Design review of the part built by this model. Coordinates are the model's own, in mm. A direction names the side the tool comes from. Give positions to 0.01 mm unless a question says otherwise; leave off trailing zeros. Loops run counter-clockwise (first coordinate to the right, second up) from the corner with the lowest first, then second, coordinate; pieces in that order, holes last.
from build123d import *

# Parameters (mm, degrees)
SKIZZE1_W                       = 21.5
SKIZZE1_H                       = 17
AUFSATZ_LINEAR_AUSTRAGEN1_DEPTH = 1
VERRUNDUNG1_R                   = 0.5
SCHNITT_LINEAR_AUSTRAGEN1_REACH = 25.141
SKIZZE4_W                       = 3
SKIZZE4_H                       = 0.25
SCHNITT_LINEAR_AUSTRAGEN2_DEPTH = 1
VERRUNDUNG2_R                   = 0.5
SCHNITT_LINEAR_AUSTRAGEN3_DEPTH = 1
SCHNITT_LINEAR_START            = -1
SCHNITT_LINEAR_AUSTRAGEN4_DEPTH = 1


with BuildPart() as part:
    # Skizze1 → Aufsatz-Linear austragen1 (new body)
    with BuildSketch(Plane(origin=(0, 0, 0), x_dir=(1, 0, 0), z_dir=(0, 1, 0))):
        Rectangle(SKIZZE1_W, SKIZZE1_H)
    extrude(amount=AUFSATZ_LINEAR_AUSTRAGEN1_DEPTH)

    # Verrundung1
    verrundung1_edges = [part.edges().sort_by_distance(p)[0] for p in [
        (-10.75, 1, 0),
        (10.75, 1, 0),
        (0, 1, -8.5),
    ]]
    fillet(verrundung1_edges, radius=VERRUNDUNG1_R)

    # Schnitt-Linear austragen1: up to this face of the body (flat: up to its plane)
    schnitt_linear_austragen1_end = Plane(part.part.faces().sort_by_distance((10.75, 0.25, 0))[0])
    # Skizze2 → Schnitt-Linear austragen1 (cut, up to the picked face)
    with BuildSketch(Plane.ZY.offset(10.75), mode=Mode.PRIVATE) as schnitt_linear_austragen1_sk1:
        Polygon((8.5, 0), (7.75, 1), (8.5, 1), align=None)
    schnitt_linear_austragen1_tool1 = split(extrude(schnitt_linear_austragen1_sk1.sketch, amount=-SCHNITT_LINEAR_AUSTRAGEN1_REACH, mode=Mode.PRIVATE), bisect_by=schnitt_linear_austragen1_end, keep=Keep.BOTH, mode=Mode.PRIVATE)
    add(schnitt_linear_austragen1_tool1.solids().sort_by(Axis((-10.75, 0.666667, 8.25), (1, 0, 0)))[0], mode=Mode.SUBTRACT)

    # Skizze4 → Schnitt-Linear austragen2 (cut)
    with BuildSketch(Plane(origin=(0, 1, 0), x_dir=(1, 0, 0), z_dir=(0, 1, 0))):
        with Locations((0, -8.125)):
            Rectangle(SKIZZE4_W, SKIZZE4_H)
    extrude(amount=-SCHNITT_LINEAR_AUSTRAGEN2_DEPTH, mode=Mode.SUBTRACT)

    # Verrundung2
    # the kernel refuses this fillet: 0.5 mm, written as the material it takes off along each edge
    with BuildSketch(Plane(origin=(-10.25, 0.5, -8), x_dir=(0, 0, -1), z_dir=(-1, 0, 0))) as verrundung2_piece_1_section:
        Polygon((0, 0), (VERRUNDUNG2_R, 0), (VERRUNDUNG2_R, -VERRUNDUNG2_R), (0, -VERRUNDUNG2_R), align=None)
    verrundung2_piece_1 = extrude(amount=VERRUNDUNG2_R, mode=Mode.PRIVATE)
    verrundung2_piece_1 = verrundung2_piece_1 - Plane(origin=(-10.25, 0.5, -8), x_dir=(0, -0.7071067811865475, 0.7071067811865475), z_dir=(-1, 0, 0)) * Sphere(VERRUNDUNG2_R, mode=Mode.PRIVATE)
    add(verrundung2_piece_1, mode=Mode.SUBTRACT)
    with BuildSketch(Plane(origin=(10.25, 0.5, -8), x_dir=(0, 0, -1), z_dir=(1, 0, 0))) as verrundung2_piece_2_section:
        Polygon((0, 0), (VERRUNDUNG2_R, 0), (VERRUNDUNG2_R, VERRUNDUNG2_R), (0, VERRUNDUNG2_R), align=None)
    verrundung2_piece_2 = extrude(amount=VERRUNDUNG2_R, mode=Mode.PRIVATE)
    verrundung2_piece_2 = verrundung2_piece_2 - Plane(origin=(10.25, 0.5, -8), x_dir=(0, -0.7071067811865475, 0.7071067811865475), z_dir=(1, 0, 0)) * Sphere(VERRUNDUNG2_R, mode=Mode.PRIVATE)
    add(verrundung2_piece_2, mode=Mode.SUBTRACT)
    with BuildSketch(Plane(origin=(10.75, -1.25, -8.5), x_dir=(0, 0, 1), z_dir=(0, 1, 0))) as verrundung2_piece_3:
        with BuildLine():
            CenterArc((VERRUNDUNG2_R, -VERRUNDUNG2_R), VERRUNDUNG2_R, 90, 90)
            Line((0, -VERRUNDUNG2_R), (0, 0))
            Line((0, 0), (VERRUNDUNG2_R, 0))
        make_face()
    extrude(amount=1.75, mode=Mode.SUBTRACT)
    with BuildSketch(Plane(origin=(-10.75, -1.25, -8.5), x_dir=(0, 0, 1), z_dir=(0, 1, 0))) as verrundung2_piece_4:
        with BuildLine():
            CenterArc((VERRUNDUNG2_R, VERRUNDUNG2_R), VERRUNDUNG2_R, 180, 90)
            Line((0, VERRUNDUNG2_R), (0, 0))
            Line((0, 0), (VERRUNDUNG2_R, 0))
        make_face()
    extrude(amount=1.75, mode=Mode.SUBTRACT)

    # Skizze5 → Schnitt-Linear austragen3 (cut)
    with BuildSketch(Plane(origin=(0, 1, 0), x_dir=(1, 0, 0), z_dir=(0, 1, 0))):
        with BuildLine():
            Line((-3.5, 5.1), (-3.5, 4.1))
            Line((-3.5, 4.1), (-1.936491673, 4.1))
            ThreePointArc((-1.936491673, 4.1), (-2, 4.6), (-1.936491673, 5.1))
            Line((-1.936491673, 5.1), (-3.5, 5.1))
        make_face()
        with BuildLine():
            ThreePointArc((1.936491673, 5.1), (0, 6.6), (-1.936491673, 5.1))
            Line((-1.936491673, 5.1), (1.936491673, 5.1))
        make_face()
        with BuildLine():
            ThreePointArc((-1.936491673, 5.1), (-2, 4.6), (-1.936491673, 4.1))
            Line((-1.936491673, 4.1), (1.936491673, 4.1))
            ThreePointArc((1.936491673, 4.1), (1.984059393, 4.347991415), (2, 4.6))
            ThreePointArc((2, 4.6), (1.984059393, 4.852008585), (1.936491673, 5.1))
            Line((1.936491673, 5.1), (-1.936491673, 5.1))
        make_face()
        with BuildLine():
            Line((1.936491673, 4.1), (-1.936491673, 4.1))
            ThreePointArc((-1.936491673, 4.1), (0, 2.6), (1.936491673, 4.1))
        make_face()
        with BuildLine():
            ThreePointArc((2, 4.6), (1.984059393, 4.347991415), (1.936491673, 4.1))
            Line((1.936491673, 4.1), (3.5, 4.1))
            Line((3.5, 4.1), (3.5, 5.1))
            Line((3.5, 5.1), (1.936491673, 5.1))
            ThreePointArc((1.936491673, 5.1), (1.984059393, 4.852008585), (2, 4.6))
        make_face()
    extrude(amount=-SCHNITT_LINEAR_AUSTRAGEN3_DEPTH, mode=Mode.SUBTRACT)

    # Skizze6 → Schnitt-Linear austragen4 (cut)
    with BuildSketch(Plane(origin=(0, 1, 0), x_dir=(1, 0, 0), z_dir=(0, 1, 0)).offset(SCHNITT_LINEAR_START)):
        with BuildLine():
            Line((1, 8.5), (1, -5.5))
            ThreePointArc((1, -5.5), (0, -6.5), (-1, -5.5))
            Line((-1, -5.5), (-1, 8.5))
            ThreePointArc((-1, 8.5), (0, 9.5), (1, 8.5))
        make_face()
    extrude(amount=SCHNITT_LINEAR_AUSTRAGEN4_DEPTH, mode=Mode.SUBTRACT)


solid = part.part
Q1. Take a section at D-D (z = -6). Give the boundary of the cut face in (x, y), plus the area to 3 significant figures.
Results:
outline: (-10.75, 0) - (-1.43, 0) - (-1.43, 1) - (-10.25, 1) arc R0.5 ccw to (-10.75, 0.5) - close; (1.43, 0) - (10.75, 0) - (10.75, 0.5) arc R0.5 ccw to (10.25, 1) - (1.43, 1) - close
area: 18.5 mm2
Q2. Tool access review of faces 1 (the face through (1.6, 0.5, -5.8)), 2 (the face through (1, 0.5, -7.4)), 3 (the face through (-2, 1, 0)): name each direction out of +Z, -Z, +X, -X, +Y, -Y from which nothing blocks a thin tool from reaching the whole face with its end or side.
Results:
face 1: +Y, -Y
face 2: -Z, +Y, -Y
face 3: +Z, -Z, +X, -X, +Y
Q3. Take a section at B-B (z = 4.25). Give the boundary of the cut face in (x, y).
Results:
outline: (-10.75, 0) - (-1, 0) - (-1, 1) - (-10.25, 1) arc R0.5 ccw to (-10.75, 0.5) - close; (1, 0) - (10.75, 0) - (10.75, 0.5) arc R0.5 ccw to (10.25, 1) - (1, 1) - close
Q4. Take a section at C-C (x = 5.5). Give the boundary of the cut face in (y, z).
Results:
outline: (0, -8.5) - (0.5, -8.5) arc R0.5 ccw to (1, -8) - (1, 7.75) - (0, 8.5) - close
Q5. Wall thickness on line 1 (X direction, y = 0.3, z = -2.75); line 2 (X direction, y = 0.35, z = -5.75); line 3 (Z direction, x = -7, y = 0.5) (3 decimals): over which ranges is each line inside the solid? List them lowest first.
Results:
line 1: x = -10.75 to -1, 1 to 10.75
line 2: x = -10.75 to -1.64, 1.64 to 10.75
line 3: z = -8.5 to 8.125
Q6. Draft analysis for pull direction X (two halves, no side actions). For faces 4 (the face through (-1.6, 0.5, -3.4)), 5 (the face through (-0.2, 0.8, 7.9)), state which applies: pulls with the +X half, pulls with the -X half, needs draft (parallel to the pull), parting line crosses it, or undercut.
Results:
face 4: undercut
face 5: needs draft
Q7. Insertion check: pin 1 (5 mm diameter, centred on x = 6.5, z = 2.5, fed in from -Y); pin 2 (0.5 mm diameter, centred on x = 0.5, y = 0.5, fed in from +Z). Each pin has a flat end and moves straight along its axis. Give the tip position at first contact, or say it passes through.
Results:
pin 1: stops at y = 0
pin 2: stops at z = 8.31
Q8. Take a section at A-A (x = 0). Give the boundary of the cut face in (y, z).
Results:
outline: (0, 6.5) - (1, 6.5) - (1, 7.75) - (0.67, 8) - (0, 8) - close; (0, 8.25) - (0.33, 8.25) - (0, 8.5) - close
